from build123d import *

# Parameters (mm, degrees)
F0_W     = 60
F0_H     = 60
F0_R     = 22.5
F1_DEPTH = 30
F2_DEPTH = 22.5
F3_R     = 22.49999
F4_R     = 29.99999


# Not quite as in the source:
# - a fillet or chamfer is up to 0.001 mm smaller than in the source, because OpenCascade refuses the exact size
# - a feature names something its author has since deleted; it is built from what else it names


with BuildPart() as f1:
    # F0 (on Top) → F1 (new body)
    with BuildSketch(Plane.XY):
        Rectangle(F0_W, F0_H)
        Circle(F0_R, mode=Mode.SUBTRACT)
        Circle(F0_R)
    extrude(amount=F1_DEPTH)

    # F0 (on Top) → F2 (cut)
    with BuildSketch(Plane.XY):
        Circle(F0_R)
    extrude(amount=F2_DEPTH, mode=Mode.SUBTRACT)

    # F3 (radius 22.5 in the source; OpenCascade refuses exactly that, so slightly less here)
    f3_edges = [f1.edges().sort_by_distance(p)[0] for p in [
        (-22.5, 0, 22.5),
    ]]
    fillet(f3_edges, radius=F3_R)

    # F4 (radius 30 in the source; OpenCascade refuses exactly that, so slightly less here)
    f4_edges = [f1.edges().sort_by_distance(p)[0] for p in [
        (0, -30, 30),
        (0, 30, 30),
    ]]
    fillet(f4_edges, radius=F4_R)


solid = f1.part
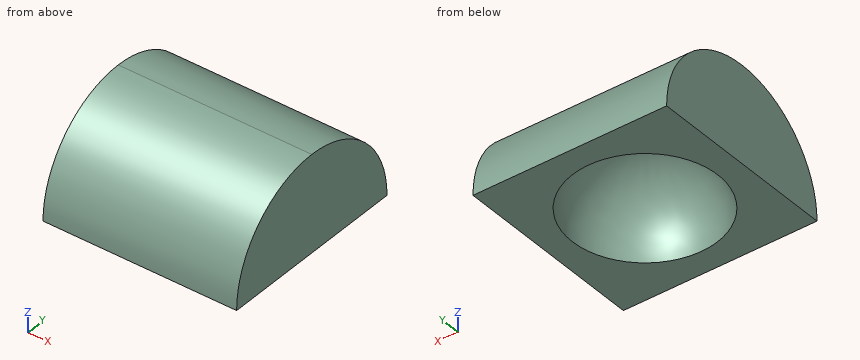
For this review, take the finished solid that the model builds, in its own axes (mm). Coordinates: 2 decimals unless noted, no trailing zeros. Loops run counter-clockwise (first coordinate to the right, second up) from the corner with the lowest first, then second, coordinate; pieces in that order, holes last. Notation, with made-up numbers: (26.25, 44.5) - (40.25, 44.5) arc R15 cw to (40.25, 49.5) - close; hole circle Ø9 at (46, 32.5). An arc over 180 degrees is marked (long way). Use a Markdown table: item, result. Add a question column.
Item 1: We need section A-A (y = -24). Give the boundary of the cut face in (x, z).
Item 2: We need section B-B (z = 25). Give the boundary of the cut face in (x, y), and give its area (3 significant figures).
Item 3: Insertion check: pin 1 Ø8 at (x, y) = (5, -9) entering from -Z; pin 2 Ø4 at (x, y) = (-6, -18.5) entering from +Z; pin 3 Ø6 at (x, z) = (11, 21) entering from +Y; pin 4 Ø10 at (y, z) = (23.5, 21) entering from +X. Each pin has a flat end and moves straight along its axis. Give the tip position at first contact, or say it passes through.
Results list:
| question | item | result |
|---|---|---|
| 1 | outline | (-30, 0) - (30, 0) - (30, 18) - (-30, 18) - close |
| 2 | outline | (-30, -16.58) - (30, -16.58) - (30, 16.58) - (-30, 16.58) - close |
| 2 | area | 1,990 mm^2 |
| 3 | pin 1 | stops at z = 17.37 |
| 3 | pin 2 | stops at z = 25.05 |
| 3 | pin 3 | stops at y = 24 |
| 3 | pin 4 | stops at x = 30 |
